```python
from build123d import *

# Parameters (mm, degrees)
F0_W     = 8
F0_H     = 8
F0_H_2   = 16
F1_DEPTH = 20.90309


with BuildPart() as f1:
    # F0 (on Front) → F1 (new body)
    with BuildSketch(Plane.XZ):
        with Locations((-20.720104, 12.105988)):
            Rectangle(F0_W, F0_H)
        with Locations((-28.720104, 12.105988)):
            Rectangle(F0_W, F0_H)
        Polygon((-32.720104, 16.105988), (-32.720104, 24.105988), (-40.720104, 24.105988), (-48.720104, 24.105988), (-48.720104, 8.105988), (-32.720104, 8.105988), align=None)
        with Locations((-36.720104, 32.105988)):
            Rectangle(F0_W, F0_H_2)
        with Locations((-44.720104, 32.105988)):
            Rectangle(F0_W, F0_H_2)
    extrude(amount=-F1_DEPTH)


solid = f1.part
```
The listing builds one solid part. Answer for the finished solid, in the listing's coordinates (mm). A direction names the side the tool comes from. Give positions to 0.01 mm unless a question says otherwise; leave off trailing zeros. Order: outer loops, then holes, each group sorted by start corner. A loop starts at its lowest first (then second) coordinate and runs counter-clockwise, first axis right, second up. Notation, with made-up numbers: (16, 12.25) -> (31, 12.25) arc R24 ccw to (31, 30.25) -> close; hole circle Ø4 at (13, 34). An arc over 180 degrees is marked (long way). Answer as a JSON object with one key per item and string values. Group by question number.
Item 1: The part is cut by section B-B on x = -32. Write down the section's boundary in (y, z), and give its area (3 significant figures).
Item 2: Flat-ended cylindrical pins translate along their axes: pin 1 (2 mm diameter, centred on y = 16, z = 28, fed in from +X); pin 2 (8 mm diameter, centred on x = -26.5, y = 11, fed in from +Z). Find the tip coordinate at first contact, or state that the pin passes through.
Item 3: Consider L1, parallel to X at y = 6.5, z = 24; L2, parallel to Z at x = -21, y = 8.25. Determine where each line is inside the solid, lowest interval first. Write a range as from..to.
Item 4: A tool of negligible diameter and unlimited length cuts with its end or side. For faces 1 (the flat face through (-48.72, 10, 24)), 2 (the flat face through (-32.72, 10, 28)), from which of +Z, -Z, +X, -X, +Y, -Y can it reach the whole face along a straight path? Write none if from no direction.
Item 5: The part is cut by section A-A on y = 9.5. Write down the section's boundary in (x, z).
Item 6: The part is cut by section C-C on z = 35. Write down the section's boundary in (x, y).
Result set:
{
 "1": {"outline": "(0, 8.11) -> (20.9, 8.11) -> (20.9, 16.11) -> (0, 16.11) -> close", "area": "167 mm²"},
 "2": {"pin 1": "x = -32.72", "pin 2": "z = 16.11"},
 "3": {"L1": "-48.72..-32.72", "L2": "8.11..16.11"},
 "4": {"face 1": "+Z, -Z, -X, +Y, -Y", "face 2": "+Z, +X, +Y, -Y"},
 "5": {"outline": "(-48.72, 8.11) -> (-16.72, 8.11) -> (-16.72, 16.11) -> (-32.72, 16.11) -> (-32.72, 40.11) -> (-48.72, 40.11) -> close"},
 "6": {"outline": "(-48.72, 0) -> (-32.72, 0) -> (-32.72, 20.9) -> (-48.72, 20.9) -> close"}
}
